Design review of the part shown in the three views and the two pictorial views. Dimensions are in mm from the part's minimum x, y and z. A direction names the side the tool comes from. Coordinates: 2 decimals unless noted, no trailing zeros. Loops run counter-clockwise (first coordinate to the right, second up) from the corner with the lowest first, then second, coordinate; pieces in that order, holes last. Notation, with made-up numbers: M 70,62 L 88,62 A21 ccw 88,78 Z; hole C 27.5,40.5 d8. An arc over 180 degrees is marked long. Use one line per item in the form item = value.
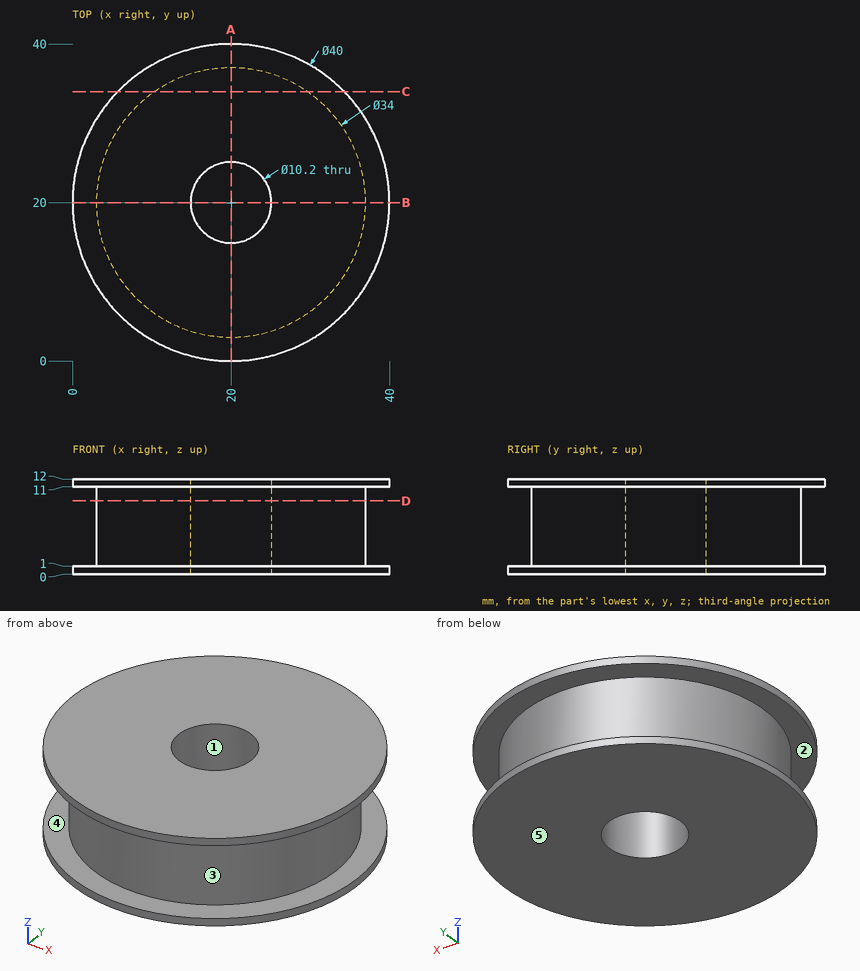
1. Add section C-C (y = 34). State the section outline as (x, z) points, then the cut area to 3 significant figures.
Response values:
outline = M 5.72,0 L 34.28,0 L 34.28,1 L 29.64,1 L 29.64,11 L 34.28,11 L 34.28,12 L 5.72,12 L 5.72,11 L 10.36,11 L 10.36,1 L 5.72,1 Z
area = 250 mm^2
2. Add section D-D (z = 9.25). State the section outline as (x, y) points, then the cut area to 3 significant figures.
Response values:
outline = C 20,20 d34; hole C 20,20 d10.2
area = 826 mm^2
3. Wall thickness on line 1 along Y through (x, z) = (20, 3.75); line 2 along X through (y, z) = (16, 8); line 3 along Z through (x, y) = (37, 23.5): over which ranges is each line inside the solid? List them lowest first. Write a range as from..to.
Response values:
line_1 = 3..14.9, 25.1..37
line_2 = 3.48..16.84, 23.16..36.52
line_3 = 0..1, 11..12
4. The part is to be moulded in two halves that separate along X. For the marked faces 1, 2 and 3, say which applies: pulls with the +X half, pulls with the -X half, needs draft (parallel to the pull), parting line crosses it, or undercut.
Response values:
face_1 = undercut
face_2 = needs draft
face_3 = parting line crosses it
5. Machinability: for the marked faces 4 and 5, which of the approach directions +Z, -Z, +X, -X, +Y, -Y give a long, thin tool a straight path to every point of the face, cutting with its end or side? Answer none if there is none.
Response values:
face_4 = none
face_5 = -Z, +X, -X, +Y, -Y
6. Add section A-A (x = 20). State the section outline as (y, z) points, then the cut area to 3 significant figures.
Response values:
outline = M 0,0 L 14.9,0 L 14.9,12 L 0,12 L 0,11 L 3,11 L 3,1 L 0,1 Z; M 25.1,0 L 40,0 L 40,1 L 37,1 L 37,11 L 40,11 L 40,12 L 25.1,12 Z
area = 298 mm^2
7. Insertion check: P1, Ø4, axis at y = 32, z = 1.5, coming from the +X side; P2, Ø2, axis at y = 23, z = 6.5, coming from the +X side; P3, Ø4, axis at y = 27.5, z = 5, coming from the +X side. Each pin has a flat end and moves straight along its axis. Give the tip position at first contact, or say it passes through.
Response values:
P1 = 37.28
P2 = 36.88
P3 = 36.09
